Verification items for the finished model (mm, model axes). A direction names the side the tool comes from. Round coordinates to 2 decimals unless told otherwise and drop trailing zeros. Order: outer loops, then holes, each group sorted by start corner. A loop starts at its lowest first (then second) coordinate and runs counter-clockwise, first axis right, second up. Notation, with made-up numbers: M -31.5,50.25 L -0.5,50.25 A19 ccw -0.5,76.25 Z; hole C 52,25.25 d2. An arc over 180 degrees is marked long. Use one line per item in the form item = value. Start each with the question number.
Item 1: Cross-section at A-A on y = 0. Enter the section's corners in (x, z).
Item 2: Cross-section at B-B on z = -1.5. Enter the section's corners in (x, y) (3 decimals), then the cut area to 3 significant figures.
Item 3: Thickness scan on probe 1 along Y at (x, z) = (-1.5, 3.25); probe 2 along Y at (x, z) = (0, 3); probe 3 along X at (y, z) = (3.5, 3). Record the ranges inside material, lowest first. Write a range as [from, to].
Item 4: Cross-section at C-C on x = -3. Enter the section's corners in (y, z).
Item 5: Release check for a two-part mould opening along Y. For faces 6 (the flat face through (6, -2.375, 0)), 7 (the flat face through (1.12, -6.69, 0.07)), 8 (the flat face through (4, 2, -5)), 9 (the cylindrical face through (7.375, 4.225, 0.07)) record: +Y half, -Y half, draft (parallel to the pull), parting line (faces both ways), or undercut.
Item 6: Tool access check on faces 1 (the flat face through (6, 2.375, 0)), 2 (the flat face through (2.221, -3.914, -0.07)), 3 (the flat face through (-5.235, 4.317, 0.07)), 4 (the flat face through (-4.5, 0, 0)), 5 (the flat face through (5.235, -4.317, 0.07)). Record the directions out of +Z, -Z, +X, -X, +Y, -Y that give a thin tool (end or side, any length) a straight path to the whole face; none if there is none.
Item 7: Go/stop test with flat-tipped pins: pin 1 Ø3 at (x, y) = (-0.5, 1) entering from -Z; pin 2 Ø4 at (y, z) = (0, -2.5) entering from +X; pin 3 Ø1.8 at (x, z) = (-7, -2) entering from +Y; pin 4 Ø2 at (y, z) = (-3.5, -0.5) entering from +X. Record where each tip stops, or that it passes through.
Item 8: Cross-section at D-D on x = 1.5. Enter the section's corners in (y, z), then the cut area to 3 significant figures.
from build123d import *

# Parameters (mm, degrees)
SKETCH1_R           = 8.5
SKETCH1_R_2         = 4
BOSS_EXTRUDE1_DEPTH = 5
SKETCH2_W           = 4.75
SKETCH2_H           = 10
CUT_EXTRUDE3_DEPTH  = 4
CIRPATTERN1_COUNT   = 6


with BuildPart() as part:
    # Sketch1 → Boss-Extrude1 (new body, symmetric)
    with BuildSketch(Plane.XY):
        Circle(SKETCH1_R)
        Circle(SKETCH1_R_2, mode=Mode.SUBTRACT)
    extrude(amount=BOSS_EXTRUDE1_DEPTH, both=True)

    # Sketch2 → Cut-Extrude3 (cut)
    with BuildSketch(Plane(origin=(-8.5, -17.193061184, 0), x_dir=(0, -1, 0), z_dir=(1, 0, 0))):
        with Locations((-17.193061184, 0)):
            Rectangle(SKETCH2_W, SKETCH2_H)
    cut_extrude3 = extrude(amount=CUT_EXTRUDE3_DEPTH, mode=Mode.SUBTRACT)

    # CirPattern1: Cut-Extrude3 ×6 about axis
    cirpattern1_axis = Axis((0, 0, 0), (0, 0, 1))
    for i in range(1, CIRPATTERN1_COUNT):
        add(cut_extrude3.rotate(cirpattern1_axis, i * 360 / CIRPATTERN1_COUNT), mode=Mode.SUBTRACT)


solid = part.part
Output values:
q1.outline = M -4.5,-5 L -4,-5 L -4,5 L -4.5,5 Z; M 4,-5 L 4.5,-5 L 4.5,5 L 4,5 Z
q2.outline = M -8.161,-2.375 A8.5 ccw -6.138,-5.881 L -4.307,-2.71 L -0.193,-5.085 L -2.024,-8.256 A8.5 ccw 2.024,-8.256 L 0.193,-5.085 L 4.307,-2.71 L 6.138,-5.881 A8.5 ccw 8.161,-2.375 L 4.5,-2.375 L 4.5,2.375 L 8.161,2.375 A8.5 ccw 6.138,5.881 L 4.307,2.71 L 0.193,5.085 L 2.024,8.256 A8.5 ccw -2.024,8.256 L -0.193,5.085 L -4.307,2.71 L -6.138,5.881 A8.5 ccw -8.161,2.375 L -4.5,2.375 L -4.5,-2.375 Z; hole C 0,0 d8
q2.area = 65.9 mm2
q3.probe_1 = [-8.37, -7.35], [-4.33, -3.71], [3.71, 4.33], [7.35, 8.37]
q3.probe_2 = [-8.5, -4], [4, 8.5]
q3.probe_3 = [-7.75, -4.76], [-2.94, -1.94], [1.94, 2.94], [4.76, 7.75]
q4.outline = M -3.46,-5 L -2.65,-5 L -2.65,5 L -3.46,5 Z; M 2.65,-5 L 3.46,-5 L 3.46,5 L 2.65,5 Z
q5.face_6 = undercut
q5.face_7 = undercut
q5.face_8 = draft
q5.face_9 = +Y half
q6.face_1 = +Z, -Z, +X
q6.face_2 = +Z, -Z
q6.face_3 = +Z, -Z, +Y
q6.face_4 = +Z, -Z, -X
q6.face_5 = +Z, -Z, -Y
q7.pin_1 = through
q7.pin_2 = 4.5
q7.pin_3 = 5.88
q7.pin_4 = 8.12
q8.outline = M -8.37,-5 L -7.35,-5 L -7.35,5 L -8.37,5 Z; M -4.33,-5 L -3.71,-5 L -3.71,5 L -4.33,5 Z; M 3.71,-5 L 4.33,-5 L 4.33,5 L 3.71,5 Z; M 7.35,-5 L 8.37,-5 L 8.37,5 L 7.35,5 Z
q8.area = 32.8 mm2
